from build123d import *

# Parameters (mm, degrees)
CROQUIS6_R              = 4.25
SALIENTE_EXTRUIR2_DEPTH = 7.25
CROQUIS7_W              = 35
CROQUIS7_H              = 35
SALIENTE_EXTRUIR3_DEPTH = 32
CHAFL_N1_SIZE           = 10
CROQUIS8_W              = 14.5
CROQUIS8_H              = 12.03
CORTAR_EXTRUIR4_DEPTH   = 30.5
CROQUIS9_W              = 5
CROQUIS9_H              = 13
CORTAR_EXTRUIR5_DEPTH   = 10
REDONDEO1_R             = 5
CROQUIS10_R             = 1.5
CORTAR_EXTRUIR6_DEPTH   = 10
CROQUIS11_R             = 2.5
CORTAR_EXTRUIR7_DEPTH   = 30


with BuildPart() as part:
    # Croquis6 → Saliente-Extruir2 (new, symmetric)
    with BuildSketch(Plane(origin=(0, 0, 0), x_dir=(0, 0, -1), z_dir=(1, 0, 0))):
        with BuildLine():
            Line((0, 17.5), (25, 17.5))
            Line((25, 17.5), (25, -17.5))
            Line((25, -17.5), (0, -17.5))
            ThreePointArc((0, -17.5), (-17.5, 0), (0, 17.5))
        make_face()
        with Locations(Location((0, 0, 0), (0, 0, 180))):
            Circle(CROQUIS6_R, mode=Mode.SUBTRACT)
    extrude(amount=SALIENTE_EXTRUIR2_DEPTH, both=True)

    # Croquis7 → Saliente-Extruir3 (add)
    with BuildSketch(Plane(origin=(0, 0, -25), x_dir=(-1, 0, 0), z_dir=(0, 0, -1))):
        Rectangle(CROQUIS7_W, CROQUIS7_H)
    extrude(amount=SALIENTE_EXTRUIR3_DEPTH)

    # Chaflán1
    chafl_n1_edges = [part.edges().sort_by_distance(p)[0] for p in [
        (-17.5, 0, -25),
        (17.5, 0, -25),
    ]]
    chamfer(chafl_n1_edges, length=CHAFL_N1_SIZE)

    # Croquis8 → Cortar-Extruir4 (cut)
    with BuildSketch(Plane(origin=(0, 0, -57), x_dir=(-1, 0, 0), z_dir=(0, 0, -1))):
        with Locations((-2.25, 0)):
            Rectangle(CROQUIS8_W, CROQUIS8_H)
    extrude(amount=-CORTAR_EXTRUIR4_DEPTH, mode=Mode.SUBTRACT)

    # Croquis9 → Cortar-Extruir5 (cut)
    with BuildSketch(Plane(origin=(17.5, 0, 0), x_dir=(0, 0, -1), z_dir=(1, 0, 0))):
        with Locations((29, 0)):
            Rectangle(CROQUIS9_W, CROQUIS9_H)
    extrude(amount=-CORTAR_EXTRUIR5_DEPTH, mode=Mode.SUBTRACT)

    # Redondeo1
    redondeo1_edges = [part.edges().sort_by_distance(p)[0] for p in [
        (-17.5, -17.5, -46),
        (-17.5, 17.5, -46),
        (17.5, 17.5, -46),
        (17.5, -17.5, -46),
    ]]
    fillet(redondeo1_edges, radius=REDONDEO1_R)

    # Croquis10 → Cortar-Extruir6 (cut)
    with BuildSketch(Plane(origin=(0, 0, -57), x_dir=(-1, 0, 0), z_dir=(0, 0, -1))):
        with Locations((-12.5, 12.5)):
            Circle(CROQUIS10_R)
        with Locations((12.5, 12.5)):
            Circle(CROQUIS10_R)
        with Locations((12.5, -12.5)):
            Circle(CROQUIS10_R)
        with Locations((-12.5, -12.5)):
            Circle(CROQUIS10_R)
    extrude(amount=-CORTAR_EXTRUIR6_DEPTH, mode=Mode.SUBTRACT)

    # Croquis11 → Cortar-Extruir7 (cut)
    with BuildSketch(Plane.XY.offset(20)):
        Circle(CROQUIS11_R)
    extrude(amount=-CORTAR_EXTRUIR7_DEPTH, mode=Mode.SUBTRACT)


solid = part.part
Read the model definition and answer for the solid it produces. Units are mm, in the model's axes. A direction names the side the tool comes from. Round coordinates to 2 decimals unless told otherwise and drop trailing zeros. Write each loop counter-clockwise with the first axis right and the second up, starting at its lowest first coordinate (ties: lowest second). Pieces come first, ordered by that corner, then holes.
1. The part is cut by section C-C, the plane z = -36. Determine the outline of the cut face in (x, y) (3 decimals), then the cut area to 3 significant figures.
2. The part is cut by section D-D, the plane x = 4. Determine the outline of the cut face in (y, z) (3 decimals), then the cut area to 3 significant figures.
3. Straight lines are drawn through the part: L1, parallel to Y at x = 12.5, z = -54; L2, parallel to Y at x = 12, z = -52; L3, parallel to X at y = 0, z = 14.5. For each, find the intervals that lie inside material, in ascending order.
4. Determine the mould class of faces 1 (the face through (-16.07, -16, -43.69)), 2 (the face through (2.385, 0.751, -6.673)), 3 (the face through (0, 17.5, -34)), 4 (the face through (9.5, 0, -44)) for opening direction Y: pulls with the +Y half, pulls with the -Y half, needs draft (parallel to the pull), parting line crosses it, or undercut.
5. The part is cut by section A-A, the plane y = 0. Determine the outline of the cut face in (x, z), then the cut area to 3 significant figures.
6. The part is cut by section B-B, the plane z = -2. Determine the outline of the cut face in (x, y), then the cut area to 3 significant figures.
7. Given pin 1 Ø1 at (y, z) = (7.5, -16) entering from +X; pin 2 Ø4 at (x, y) = (0, 0) entering from -Z; pin 3 Ø4 at (x, y) = (0, -1) entering from +Z, each flat-ended and moving along its own axis, determine where each tip first touches the part or whether it passes through.
8. Which of the six approach directions +Z, -Z, +X, -X, +Y, -Y give full straight-line access (tool end or side, diameter ignored) to faces 5 (the face through (14, 12.57, -52.07)), 6 (the face through (0, 0, -10)), 7 (the face through (-7.25, 0, -9))?
Values:
1. outline: (-17.5, -12.5) arc R5 ccw to (-12.5, -17.5) - (12.5, -17.5) arc R5 ccw to (17.5, -12.5) - (17.5, 12.5) arc R5 ccw to (12.5, 17.5) - (-12.5, 17.5) arc R5 ccw to (-17.5, 12.5) - close; hole (-5, -6.015) - (9.5, -6.015) - (9.5, 6.015) - (-5, 6.015) - close
1. area: 1,030 mm2
2. outline: (-17.5, -57) - (-6.015, -57) - (-6.015, -26.5) - (6.015, -26.5) - (6.015, -57) - (17.5, -57) - (17.5, 0) arc R17.5 ccw to (-17.5, 0) - close; hole circle Ø8.5 at (0, 0)
2. area: 2,050 mm2
3. L1: y = -17.5 to -14, -11 to 11, 14 to 17.5
3. L2: y = -17.5 to -13.91, -11.09 to 11.09, 13.91 to 17.5
3. L3: x = -7.25 to -2.5, 2.5 to 7.25
4. face 1: pulls with the -Y half
4. face 2: undercut
4. face 3: pulls with the +Y half
4. face 4: undercut
5. outline: (-17.5, -57) - (-5, -57) - (-5, -26.5) - (9, -26.5) - (7.5, -25) - (7.25, -25) - (7.25, -4.25) - (2.5, -4.25) - (2.5, -10) - (-2.5, -10) - (-2.5, -4.25) - (-7.25, -4.25) - (-7.25, -25) - (-7.5, -25) - (-17.5, -35) - close; (-7.25, 4.25) - (-2.5, 4.25) - (-2.5, 17.5) - (-7.25, 17.5) - close; (2.5, 4.25) - (7.25, 4.25) - (7.25, 17.5) - (2.5, 17.5) - close; (9.5, -57) - (17.5, -57) - (17.5, -35) - (14, -31.5) - (9.5, -31.5) - close
5. area: 966 mm2
6. outline: (-7.25, -17.5) - (7.25, -17.5) - (7.25, -3.75) - (-7.25, -3.75) - close; (-7.25, 3.75) - (7.25, 3.75) - (7.25, 17.5) - (-7.25, 17.5) - close
6. area: 399 mm2
7. pin 1: stops at x = 7.25
7. pin 2: stops at z = -26.5
7. pin 3: stops at z = 17.42
8. face 5: -Z
8. face 6: +Z
8. face 7: +Z, -X, +Y, -Y
